Autodesk Inventor part; units mm, degrees
ref_plane "YZ Plane" through (0, 0, 0) normal (1, 0, 0) x (0, 1, 0)
ref_plane "XZ Plane" through (0, 0, 0) normal (0, 1, 0) x (-1, 0, 0)
ref_plane "XY Plane" through (0, 0, 0) normal (0, 0, 1) x (1, 0, 0)
sketch "Sketch1" plane through (0, 0, 0) normal (0, 0, 1) x (1, 0, 0)
  line L0 (-15.875, -4.7625) -> (15.875, -4.7625)
  line L1 (15.875, -4.7625) -> (15.875, 4.7625)
  line L2 (15.875, 4.7625) -> (-15.875, 4.7625)
  line L3 (-15.875, 4.7625) -> (-15.875, -4.7625)
  line L4 (-15.875, -4.7625) -> (15.875, 4.7625) construction
  point P0 (0, 0)
  point P1 (0, 0)
  dimension "d0" = 9.525
  dimension "d1" = 31.75
extrude "Extrusion1" add sketch "Sketch1" along normal blind 1.6256
sketch "Sketch2" plane through (0, 0, 1.6256) normal (0, 0, 1) x (1, 0, 0)
  line L0 (-22.225, 0) -> (22.225, 0) construction
  line L1 (0, -6.6675) -> (0, 6.6675) construction
  point P0 (0, 0)
  point P1 (-12.7, 0)
  point P2 (12.7, 0)
  dimension "d4" = 25.4
hole "Hole1" at (-12.7, 0, 1.6256) at (12.7, 0, 1.6256) direction (0, 0, -1) diameter 2.4384 end through all
sketch "Sketch3" plane through (0, 0, 1.6256) normal (0, 0, 1) x (1, 0, 0)
  line L0 (-22.225, 0) -> (22.225, 0) construction
  line L1 (0, -6.6675) -> (0, 6.6675) construction
  point P0 (0, 0)
  point P1 (-6.35, 0)
  point P2 (6.35, 0)
  dimension "d12" = 12.7
hole "Hole2" at (-6.35, 0, 1.6256) at (6.35, 0, 1.6256) direction (0, 0, -1) diameter 2.286 end through all
properties part number "J002609"
Could you check a few things on this model? Use its own coordinates, in mm. Round coordinates to 2 decimals unless told otherwise and drop trailing zeros. Order: outer loops, then holes, each group sorted by start corner. A loop starts at its lowest first (then second) coordinate and runs counter-clockwise, first axis right, second up. Notation, with made-up numbers: M -33.75,2 L -20.75,2 A11 cw -20.75,8 Z; hole C 2.25,-26 d10. An arc over 180 degrees is marked long. One line per question, with ' | ' between items. Start each with the question number.
(1) Suppose I cut it at A-A on x = -6.35. List the corners of the cut face in (y, z) for me, then the cut area to 3 significant figures.
(2) Suppose I cut it at B-B on z = 1.3. Count the separate pieces of the cut face and the enclosed holes in it, then the cut area to 3 significant figures.
(3) Please list where these lines run through material, in increasing order: line 1 along X through (y, z) = (-0.75, 0.7) (3 decimals); line 2 along X through (y, z) = (0, 1) (3 decimals); line 3 along Y through (x, z) = (13.5, 0.7).
(4) Thinking about a two-plate mould opening in Y: for faces 1 (the face through (0, -4.762, 1)), 2 (the face through (-12, -1, 1)), 3 (the face through (-7.314, -0.614, 0.801)), 4 (the face through (15.875, 0, 1)), which applies, +Y half, -Y half, draft (parallel to the pull), parting line (faces both ways), or undercut?
(5) For P1, Ø3, axis at x = -12.7, y = 0, coming from the -Z side, with a flat end and sliding along its axis, tell me the tip position at first contact or that it passes through.
(6) Suppose I cut it at C-C on x = -12.7. List the corners of the cut face in (y, z) for me.
Geometry results:
1) outline: M -4.76,0 L -1.14,0 L -1.14,1.63 L -4.76,1.63 Z; M 1.14,0 L 4.76,0 L 4.76,1.63 L 1.14,1.63 Z | area: 11.8 mm²
2) separate pieces: 1 | enclosed holes: 4 | area: 285 mm²
3) line 1: -15.875 to -13.661, -11.739 to -7.213, -5.487 to 5.487, 7.213 to 11.739, 13.661 to 15.875 | line 2: -15.875 to -13.919, -11.481 to -7.493, -5.207 to 5.207, 7.493 to 11.481, 13.919 to 15.875 | line 3: -4.76 to -0.92, 0.92 to 4.76
4) face 1: -Y half | face 2: undercut | face 3: undercut | face 4: draft
5) P1: z = 0
6) outline: M -4.76,0 L -1.22,0 L -1.22,1.63 L -4.76,1.63 Z; M 1.22,0 L 4.76,0 L 4.76,1.63 L 1.22,1.63 Z
